Answer from the drawing. Dimensions are ordinates in mm from the lowest x, y and z of the part. Give positions to 0.01 mm unless a question says otherwise; leave off trailing zeros. Write each loop counter-clockwise with the first axis right and the second up, starting at its lowest first coordinate (ties: lowest second). Pieces come first, ordered by that corner, then holes. Notation, with made-up numbers: (81, -19) - (103, -19) arc R19 ccw to (103, 11) - close; hole circle Ø1 at (62.5, 88). An arc over 180 degrees is marked (long way). Write item = value, one per line.
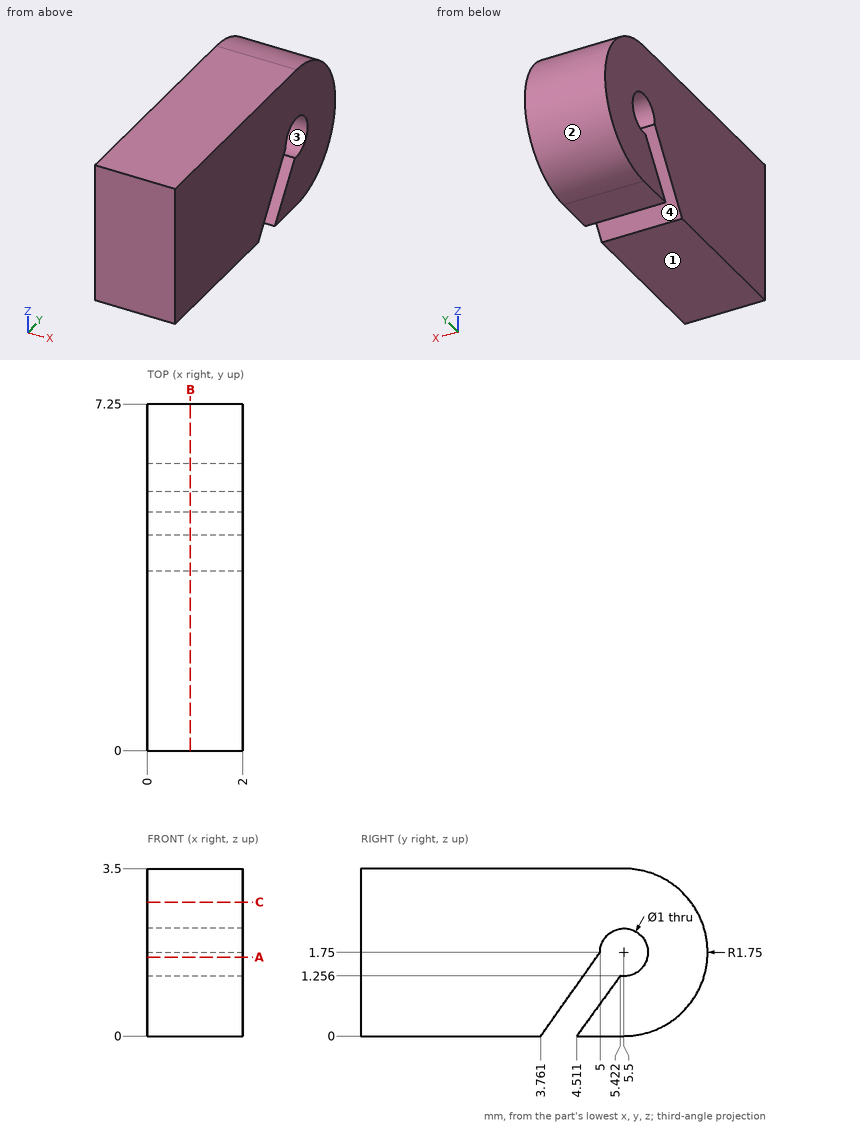
1. Given pin 1 (0.8 mm diameter, centred on y = 5.5, z = 1.75, fed in from +X); pin 2 (1 mm diameter, centred on x = 0.5, z = 2.5, fed in from +Y), each flat-ended and moving along its own axis, determine where each tip first touches the part or whether it passes through.
Solution:
pin_1 = through
pin_2 = 7.23
2. Find section C-C, the plane z = 2.8. Give the vertices of the cut face in (x, y).
Solution:
outline = (0, 0) - (2, 0) - (2, 6.9) - (0, 6.9) - close
3. Straight lines are drawn through the part: line 1 (Y direction, x = 1.95, z = 1.8); line 2 (Z direction, x = 0.8, y = 5.75) (1 decimal); line 3 (Y direction, x = 1, z = 1.65) (1 decimal). For each, find the intervals that lie inside material, in ascending order.
Solution:
line_1 = 0 to 5, 6 to 7.25
line_2 = 0 to 1.3, 2.2 to 3.5
line_3 = 0 to 4.9, 6 to 7.2
4. For a pull along Y with two mould halves and no side action, classify the marked faces 1, 2, 3 and 4 as pulls with the +Y half, pulls with the -Y half, needs draft (parallel to the pull), parting line crosses it, or undercut.
Solution:
face_1 = needs draft
face_2 = pulls with the +Y half
face_3 = undercut
face_4 = undercut
5. Find section B-B, the plane x = 0.9. Give the vertices of the cut face in (y, z).
Solution:
outline = (0, 0) - (3.76, 0) - (5, 1.75) arc R0.5 cw (long way) to (5.42, 1.26) - (4.51, 0) - (5.5, 0) arc R1.75 ccw to (5.5, 3.5) - (0, 3.5) - close
6. Find section A-A, the plane z = 1.65. Give the vertices of the cut face in (x, y).
Solution:
outline = (0, 0) - (2, 0) - (2, 4.93) - (0, 4.93) - close; (0, 5.99) - (2, 5.99) - (2, 7.25) - (0, 7.25) - close
